Could you check a few things on this model? Use its own coordinates, in mm. Face numbers are marked on the shaded views. A direction names the side the tool comes from. Coordinates: 2 decimals unless noted, no trailing zeros. Loops run counter-clockwise (first coordinate to the right, second up) from the corner with the lowest first, then second, coordinate; pieces in that order, holes last. Notation, with made-up numbers: M 81.5,1 L 109.5,1 A25 cw 109.5,34 Z; hole C 11.25,70.25 d9. An arc over 180 degrees is marked long. Write each question's results on one line, items separated by ' | '.
Autodesk Inventor part; units mm, degrees
ref_plane "YZ Plane" through (0, 0, 0) normal (1, 0, 0) x (0, 1, 0)
ref_plane "XZ Plane" through (0, 0, 0) normal (0, 1, 0) x (-1, 0, 0)
ref_plane "XY Plane" through (0, 0, 0) normal (0, 0, 1) x (1, 0, 0)
sketch "Boceto1" plane through (0, 0, 0) normal (0, 1, 0) x (-1, 0, 0)
  line L0 (105, 90) -> (-105, 90)
  line L1 (-105, 90) -> (-105, -90)
  line L2 (-105, -90) -> (105, -90)
  line L3 (105, -90) -> (105, 90)
  line L4 (105, 90) -> (-105, -90) construction
  line L5 (-105, 90) -> (105, -90) construction
  point P0 (0, 0)
  dimension "d0" = 210
  dimension "d1" = 180
extrude "Extrusión1" add sketch "Boceto1" along normal blind 20
sketch "Boceto2" plane through (0, 20, 0) normal (0, 1, 0) x (1, 0, 0)
  line L0 (-105.0239, -70) -> (104.9761, -70)
  line L1 (-105.0239, -70) -> (104.9761, -70)
  circle A0 centre (-11.5239, -50) radius 3
  circle A1 centre (11.4761, -50) radius 3
  circle A2 centre (-11.5239, -20) radius 3
  circle A3 centre (11.4761, -20) radius 3
  line L2 (-105, -90) -> (105, -90)
  circle A4 centre (28, 59) radius 3.5
  circle A5 centre (-28, 59) radius 3.5
  line L3 (105, 90) -> (-105, 90)
  line L4 (0, 90) -> (0, 53.0386)
  point P0 (0, 0)
  point P1 (0, -225)
  point P2 (0, -225)
  dimension "d4" = 20
  dimension "d5" = 20
  dimension "d6" = 30
  dimension "d7" = 30
  dimension "d8" = 20
  dimension "d9" = 7
  dimension "d11" = 7
  dimension "d12" = 31
  dimension "d13" = 31
  dimension "d14" = 28
  dimension "d15" = 28
extrude "Extrusión2" cut sketch "Boceto2" against normal blind 20 contours A0 | A1 | A2 | A3
sketch "Boceto3" plane through (0, 20, 0) normal (0, 1, 0) x (1, 0, 0)
  line L0 (105, 90) -> (-105, 90)
  line L1 (0, 90) -> (0, 58.0056)
  circle A0 centre (-28, 59) radius 3.5
  line L2 (-42, -1) -> (42, -1)
  line L3 (42, -1) -> (42, 40)
  line L4 (42, 40) -> (-42, 40)
  line L5 (-42, 40) -> (-42, -1)
  line L6 (-42, -1) -> (42, 40) construction
  line L7 (42, -1) -> (-42, 40) construction
  circle A1 centre (-11.5239, -20) radius 3
  line L8 (-37, 4) -> (37, 4)
  line L9 (37, 4) -> (37, 35)
  line L10 (37, 35) -> (-37, 35)
  line L11 (-37, 35) -> (-37, 4)
  line L12 (-37, 4) -> (37, 35) construction
  line L13 (37, 4) -> (-37, 35) construction
  point P0 (0, 0)
  point P1 (-24.876, 34.9118)
  point P2 (0, 74.0028)
  point P3 (0, 19.5)
  dimension "d23" = 84
  dimension "d24" = 41
  dimension "d25" = 19
  dimension "d26" = 74
  dimension "d27" = 31
extrude "Extrusión3" add sketch "Boceto3" along normal blind 30 contours L5 L4 L3 L2
sketch "Boceto4" plane through (0, 20, 0) normal (0, 1, 0) x (1, 0, 0)
  circle A0 centre (-56.75, 68.25) radius 1.75
  line L0 (105, 90) -> (-105, 90)
  line L1 (-55, 60) -> (-65, 60)
  line L2 (-65, 60) -> (-65, 70)
  line L3 (-65, 70) -> (-55, 70)
  line L4 (-55, 70) -> (-55, 60)
  line L5 (-55, 60) -> (-65, 70) construction
  line L6 (-65, 60) -> (-55, 70) construction
  line L7 (-105, 90) -> (-105, -90)
  circle A1 centre (-63.25, 61.75) radius 1.75
  line L8 (0, 90) -> (0, 77.3124)
  circle A2 centre (56.75, 68.25) radius 1.75
  line L9 (55, 60) -> (65, 60)
  line L10 (65, 60) -> (65, 70)
  line L11 (65, 70) -> (55, 70)
  line L12 (55, 70) -> (55, 60)
  line L13 (55, 60) -> (65, 70) construction
  line L14 (65, 60) -> (55, 70) construction
  circle A3 centre (63.25, 61.75) radius 1.75
  point P0 (0, 0)
  point P1 (-65, 65)
  point P2 (65, 65)
  dimension "d30" = 3.5
  dimension "d32" = 40
  dimension "d33" = 1.75
  dimension "d34" = 1.75
  dimension "d35" = 1.75
  dimension "d36" = 1.75
  dimension "d37" = 10
  dimension "d38" = 10
  dimension "d39" = 20
hole "Agujero1" at (-63.25, 20, -61.75) at (-56.75, 20, -68.25) at (56.75, 20, -68.25) at (63.25, 20, -61.75) direction (0, -1, 0) diameter 3.5 end through all
sketch "Boceto5" plane through (0, 20, 0) normal (0, 1, 0) x (1, 0, 0)
  circle A0 centre (56.75, 68.25) radius 1.75
  line L0 (55, 68.25) -> (55, 90.0503)
  circle A1 centre (63.25, 61.75) radius 1.75
  line L1 (65, 61.75) -> (65, 90)
  line L2 (105, 90) -> (-105, 90)
  line L3 (55, 90.0503) -> (45.0001, 90)
  line L4 (65, 90) -> (75, 90)
  line L5 (45.0001, 90) -> (75, 90)
  line L6 (75, 90) -> (75, 50)
  line L7 (75, 50) -> (45.0001, 50)
  line L8 (45.0001, 50) -> (45.0001, 90)
  line L9 (0, 90) -> (0, 68.25)
  circle A2 centre (-56.75, 68.25) radius 1.75
  line L10 (-55, 68.25) -> (-55, 90.0503)
  circle A3 centre (-63.25, 61.75) radius 1.75
  line L11 (-65, 61.75) -> (-65, 90)
  line L12 (-105, 90) -> (105, 90)
  line L13 (-55, 90.0503) -> (-45.0001, 90)
  line L14 (-65, 90) -> (-75, 90)
  line L15 (-45.0001, 90) -> (-75, 90)
  line L16 (-75, 90) -> (-75, 50)
  line L17 (-75, 50) -> (-45.0001, 50)
  line L18 (-45.0001, 50) -> (-45.0001, 90)
  point P0 (0, 0)
  dimension "d47" = 10
  dimension "d48" = 10
  dimension "d49" = 40
extrude "Extrusión4" cut sketch "Boceto5" against normal blind 10 contours A0 | A1 | L2 L6 L7 L8 | L18 L17 L16 L2
sketch "Boceto6" plane through (0, 20, 0) normal (0, 1, 0) x (1, 0, 0)
  circle A0 centre (-11.5239, -20) radius 3
  circle A1 centre (11.4761, -20) radius 3
  line L0 (-105, -90) -> (105, -90)
  line L1 (-105.0239, -70) -> (104.9761, -70)
  line L2 (-105.0239, -70) -> (104.9761, -70)
  circle A2 centre (-11.5239, -50) radius 3
  circle A3 centre (11.4761, -50) radius 3
  line L3 (-11.5239, -20) -> (11.4761, -50)
  line L4 (-11.5239, -50) -> (11.4761, -20)
  line L5 (-105, -90) -> (105, -90)
  line L6 (105, -90) -> (95.8154, -90)
  line L7 (-0.0239, -35) -> (34.9761, -35)
  line L8 (-0.0239, -35) -> (-35.0239, -35)
  line L9 (-35.0239, -35) -> (-35.0239, -70)
  line L10 (105, -70) -> (-105, -70)
  line L11 (-35.0239, -70) -> (34.9761, -70)
  line L12 (34.9761, -70) -> (34.9761, -1)
  line L13 (34.9761, -1) -> (-35.0239, -1)
  line L14 (-35.0239, -1) -> (-35.0239, -70)
  line L15 (105, -80) -> (94.0798, -80)
  line L16 (-105, -90) -> (105, -90)
  line L17 (-105, -70) -> (105, -70)
  line L18 (105, -70) -> (105, -90)
  line L19 (105, -90) -> (-105, -90)
  line L20 (-105, -90) -> (-105, -70)
  point P0 (0, 0)
  point P1 (0, -80)
  point P2 (-0.0478, -70)
  point P3 (105, -90)
  dimension "d52" = 20
  dimension "d53" = 20
  dimension "d54" = 30
  dimension "d55" = 30
  dimension "d56" = 20
  dimension "d57" = 35
  dimension "d58" = 35
  dimension "d59" = 69
extrude "Extrusión5" cut sketch "Boceto6" against normal blind 10
sketch "Boceto7" plane through (0, 20, 0) normal (0, 1, 0) x (1, 0, 0)
  circle A0 centre (-56.75, 68.25) radius 1.75
  line L0 (-56.75, 66.5) -> (-56.75, 61.75)
  circle A1 centre (-63.25, 61.75) radius 1.75
  line L1 (-56.75, 68.25) -> (-63.25, 61.75)
  point P0 (0, 0)
properties part number "base_front"
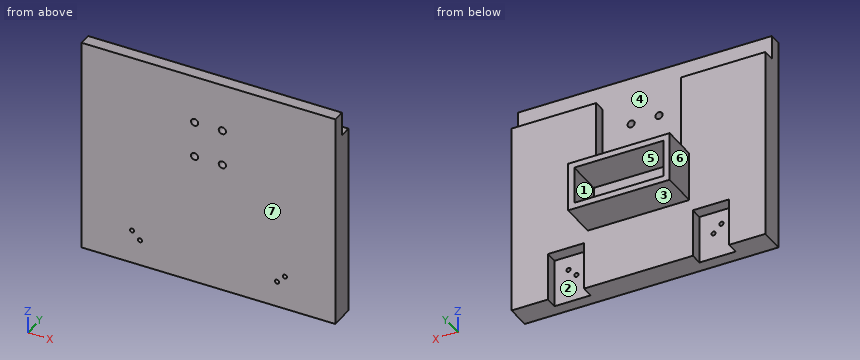
(1) If we mould it in two halves opening along X, with no side actions, what happens to the marked faces 4, 5, 6 and 7? For each: released by +X, released by -X, zero draft, split by the parting line, or undercut.
Reported:
face 4: undercut | face 5: undercut | face 6: released by -X | face 7: zero draft
(2) Imagine slicing it at D-D, the plane x = 24.5. List the corners of the cut face in (y, z) for me, and give its area (3 significant figures).
Reported:
outline: M 0,-90 L 20,-90 L 20,-40 L 50,-40 L 50,-35 L 20,-35 L 20,-4 L 50,-4 L 50,1 L 10,1 L 10,90 L 0,90 Z | area: 3,010 mm2
(3) Imagine slicing it at B-B, the plane z = -31. List the corners of the cut face in (x, y) for me.
Reported:
outline: M -105,0 L 105,0 L 105,20 L 42,20 L 42,50 L 37,50 L 37,20 L -37,20 L -37,50 L -42,50 L -42,20 L -105,20 Z
(4) Which directions (+Z, -Z, +X, -X, +Y, -Y) give clear straight access to the entire face, cutting with the end or side of a thin tool? Please do the marked faces 1, 2 and 3.
Reported:
face 1: +Y | face 2: -Z, +Y | face 3: -Z, +X, -X, +Y
(5) Imagine slicing it at C-C, the plane y = 41.5. List the corners of the cut face in (x, z) for me, and give its area (3 significant figures).
Reported:
outline: M -42,-40 L 42,-40 L 42,1 L -42,1 Z; hole M -37,-35 L 37,-35 L 37,-4 L -37,-4 Z | area: 1,150 mm2
(6) Will these pins go through, and if not, where does the flat tip stop? P1, Ø8, axis at y = 22, z = -37, coming from the -X side; P2, Ø3, axis at x = 65.5, y = 14, coming from the +Z side; P3, Ø15, axis at y = 31, z = -19, coming from the -X side; P4, Ø7, axis at x = -11.52, z = 20, coming from the +Y side.
Reported:
P1: stops at x = -105 | P2: stops at z = 70 | P3: stops at x = -42 | P4: stops at y = 10
(7) Please list where these lines run through material, in increasing order: probe 1 along X at (y, z) = (8, -68); probe 2 along X at (y, z) = (7.75, 50); probe 3 along Z at (x, y) = (-63, 4). Write a range as from..to.
Reported:
probe 1: x = -105..-58.48, -55.02..55.02, 58.48..105 | probe 2: x = -105..-14.52, -8.52..8.48, 14.48..105 | probe 3: z = -90..-63.48, -60.02..90
(8) Imagine slicing it at A-A, the plane z = 50. List the corners of the cut face in (x, y) for me.
Reported:
outline: M -105,0 L -14.52,0 L -14.52,10 L -35.02,10 L -35.02,20 L -105,20 Z; M -8.52,0 L 8.48,0 L 8.48,10 L -8.52,10 Z; M 14.48,0 L 105,0 L 105,20 L 34.98,20 L 34.98,10 L 14.48,10 Z
